The listing builds one solid part. Answer for the finished solid, in the listing's coordinates (mm). Face numbers are marked on the shaded views. A direction names the side the tool comes from. Round coordinates to 2 decimals unless told otherwise and drop trailing zeros. Loops run counter-clockwise (first coordinate to the right, second up) from the corner with the lowest first, then second, coordinate; pieces in that order, holes last. Notation, with made-up numbers: (1, 67.5) -> (45, 67.5) arc R35 ccw to (45, 106.5) -> close; hole circle Ø11 at (23, -8). An arc over 180 degrees is marked (long way). One line per question, with ' | ' between items.
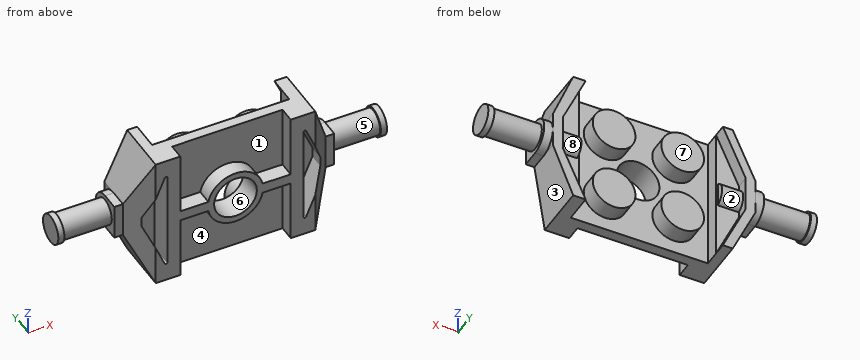
from build123d import *

# Parameters (mm, degrees)
SKETCH1_W                = 23.5
SKETCH1_H                = 15.8
BOSS_EXTRUDE1_DEPTH      = 6.3
SKETCH3_W                = 15.9
SKETCH3_H                = 15.8
CUT_EXTRUDE1_DEPTH       = 3.3
CUT_EXTRUDE2_DEPTH       = 30.009998276
CUT_EXTRUDE3_DEPTH       = 1.5
CUT_EXTRUDE4_DEPTH       = 30.009998276
BOSS_EXTRUDE2_DEPTH      = 1
BOSS_EXTRUDE3_DEPTH      = 5.6
BOSS_EXTRUDE3_DEPTH_BACK = 4.6
SKETCH9_R                = 1.5
BOSS_EXTRUDE4_START      = 1
BOSS_EXTRUDE4_DEPTH      = 1
BOSS_EXTRUDE5_DEPTH      = 5.6
BOSS_EXTRUDE5_DEPTH_BACK = 4.6
SKETCH11_R               = 1.5
CUT_EXTRUDE5_DEPTH       = 1.8
SKETCH13_R               = 2.475
CUT_EXTRUDE6_DEPTH       = 35.573689418
CUT_EXTRUDE7_DEPTH       = 2.8
SKETCH15_R               = 1.7
BOSS_EXTRUDE7_DEPTH      = 0.7
BOSS_EXTRUDE8_START      = 0.7
SKETCH16_R               = 1.7
BOSS_EXTRUDE8_DEPTH      = 0.7
SKETCH17_R               = 2.475
BOSS_EXTRUDE9_DEPTH      = 2


with BuildPart() as part:
    # Sketch1 → Boss-Extrude1 (new body)
    with BuildSketch(Plane(origin=(0, 0, 0), x_dir=(1, 0, 0), z_dir=(0, 1, 0))):
        with Locations((11.75, -7.9)):
            Rectangle(SKETCH1_W, SKETCH1_H)
    extrude(amount=BOSS_EXTRUDE1_DEPTH)

    # Sketch3 → Cut-Extrude1 (cut)
    with BuildSketch(Plane(origin=(0, 6.3, 0), x_dir=(1, 0, 0), z_dir=(0, 1, 0))):
        with Locations((11.75, -7.9)):
            Rectangle(SKETCH3_W, SKETCH3_H)
    extrude(amount=-CUT_EXTRUDE1_DEPTH, mode=Mode.SUBTRACT)

    # Sketch4 → Cut-Extrude2 (cut, through all)
    with BuildSketch(Plane(origin=(0, 6.3, 0), x_dir=(1, 0, 0), z_dir=(0, 1, 0))):
        Polygon((21.15, 0), (23.5, -5.85), (23.5, 0), align=None)
        Polygon((21.15, -15.8), (23.5, -9.95), (23.5, -15.8), align=None)
        Polygon((2.65, -15.8), (0, -9.95), (0, -15.8), align=None)
        Polygon((0, 0), (0, -5.85), (2.65, 0), align=None)
    extrude(amount=-CUT_EXTRUDE2_DEPTH, mode=Mode.SUBTRACT)

    # Sketch5 → Cut-Extrude3 (cut)
    with BuildSketch(Plane(origin=(0, 6.3, 0), x_dir=(1, 0, 0), z_dir=(0, 1, 0))):
        Polygon((3.8, 0), (1.15, -5.85), (1.15, -9.95), (3.8, -15.8), align=None)
        Polygon((19.7, 0), (19.7, -15.8), (22.35, -9.95), (22.35, -5.85), align=None)
    extrude(amount=-CUT_EXTRUDE3_DEPTH, mode=Mode.SUBTRACT)

    # Sketch7 → Cut-Extrude4 (cut, through all)
    with BuildSketch(Plane.XY.offset(15.8)):
        Polygon((0, 0), (0, 2.2), (2.65, 0), align=None)
        Polygon((21.15, 0), (23.5, 0), (23.5, 2.2), align=None)
    extrude(amount=-CUT_EXTRUDE4_DEPTH, mode=Mode.SUBTRACT)

    # Sketch8 → Boss-Extrude2 (add)
    with BuildSketch(Plane(origin=(23.5, 0, 0), x_dir=(0, 0, -1), z_dir=(1, 0, 0))):
        with BuildLine():
            Line((-9.95, 4.25), (-9.95, 2.2))
            Line((-9.95, 2.2), (-5.85, 2.2))
            Line((-5.85, 2.2), (-5.85, 4.25))
            ThreePointArc((-5.85, 4.25), (-7.9, 6.3), (-9.95, 4.25))
        make_face()
    extrude(amount=BOSS_EXTRUDE2_DEPTH)

    # Sketch9 → Boss-Extrude3 (add, two sides: drawn at the far end of the back side and taken through both)
    with BuildSketch(Plane(origin=(24.5, 0, 0), x_dir=(0, 0, -1), z_dir=(1, 0, 0)).offset(-BOSS_EXTRUDE3_DEPTH_BACK)):
        with Locations((-7.9, 4.25)):
            Circle(SKETCH9_R)
    extrude(amount=BOSS_EXTRUDE3_DEPTH + BOSS_EXTRUDE3_DEPTH_BACK)

    # Sketch10 → Boss-Extrude4 (add)
    with BuildSketch(Plane.ZY.offset(BOSS_EXTRUDE4_START)):
        with BuildLine():
            Line((5.85, 2.2), (9.95, 2.2))
            Line((9.95, 2.2), (9.95, 4.25))
            ThreePointArc((9.95, 4.25), (7.9, 6.3), (5.85, 4.25))
            Line((5.85, 4.25), (5.85, 2.2))
        make_face()
    extrude(amount=-BOSS_EXTRUDE4_DEPTH)

    # Sketch11 → Boss-Extrude5 (add, two sides: drawn at the far end of the back side and taken through both)
    with BuildSketch(Plane.ZY.offset(1).offset(-BOSS_EXTRUDE5_DEPTH_BACK)):
        with Locations(Location((7.9, 4.25, 0), (0, 0, 180))):
            Circle(SKETCH11_R)
    extrude(amount=BOSS_EXTRUDE5_DEPTH + BOSS_EXTRUDE5_DEPTH_BACK)

    # Sketch12 → Cut-Extrude5 (cut)
    with BuildSketch(Plane.XZ):
        with BuildLine():
            Line((18.3, 15.8), (5.5, 15.8))
            Line((5.5, 15.8), (5.5, 8.5))
            Line((5.5, 8.5), (8.756753271, 8.5))
            ThreePointArc((8.756753271, 8.5), (11.885259229, 11.099966048), (15.037585601, 8.528932905))
            Line((15.037585601, 8.528932905), (18.3, 8.5))
            Line((18.3, 8.5), (18.3, 15.8))
        make_face()
        with BuildLine():
            Line((8.756753271, 7.3), (5.5, 7.3))
            Line((5.5, 7.3), (5.5, 0))
            Line((5.5, 0), (18.3, 0))
            Line((18.3, 0), (18.3, 7.3))
            Line((18.3, 7.3), (15.043246729, 7.3))
            ThreePointArc((15.043246729, 7.3), (11.9, 4.7), (8.756753271, 7.3))
        make_face()
    extrude(amount=-CUT_EXTRUDE5_DEPTH, mode=Mode.SUBTRACT)

    # Sketch13 → Cut-Extrude6 (cut, through all)
    with BuildSketch(Plane.XZ):
        with Locations(Location((11.9, 7.9, 0), (0, 0, 270))):
            Circle(SKETCH13_R)
    extrude(amount=-CUT_EXTRUDE6_DEPTH, mode=Mode.SUBTRACT)

    # Sketch14 → Cut-Extrude7 (cut)
    with BuildSketch(Plane.XZ):
        with BuildLine():
            Line((4, 13.567291996), (4, 2.232708004))
            ThreePointArc((4, 2.232708004), (3.880084058, 2.085755802), (3.712067341, 2.173762423))
            Line((3.712067341, 2.173762423), (1.5, 7.35))
            Line((1.5, 7.35), (1.5, 8.45))
            Line((1.5, 8.45), (3.712067341, 13.626237577))
            ThreePointArc((3.712067341, 13.626237577), (3.880084058, 13.714244198), (4, 13.567291996))
        make_face()
        with BuildLine():
            Line((20.087932659, 2.173762423), (22.3, 7.35))
            Line((22.3, 7.35), (22.3, 8.45))
            Line((22.3, 8.45), (20.087932659, 13.626237577))
            ThreePointArc((20.087932659, 13.626237577), (19.919915942, 13.714244198), (19.8, 13.567291996))
            Line((19.8, 13.567291996), (19.8, 2.232708004))
            ThreePointArc((19.8, 2.232708004), (19.919915942, 2.085755802), (20.087932659, 2.173762423))
        make_face()
    extrude(amount=-CUT_EXTRUDE7_DEPTH, mode=Mode.SUBTRACT)

    # Sketch15 → Boss-Extrude7 (add)
    with BuildSketch(Plane.ZY.offset(6.6)):
        with Locations((7.9, 4.25)):
            Circle(SKETCH15_R)
    extrude(amount=BOSS_EXTRUDE7_DEPTH)

    # Sketch16 → Boss-Extrude8 (add)
    with BuildSketch(Plane(origin=(30.1, 0, 0), x_dir=(0, 0, -1), z_dir=(1, 0, 0)).offset(BOSS_EXTRUDE8_START)):
        with Locations(Location((-7.9, 4.25, 0), (0, 0, 180))):
            Circle(SKETCH16_R)
    extrude(amount=-BOSS_EXTRUDE8_DEPTH)

    # Sketch17 → Boss-Extrude9 (add)
    with BuildSketch(Plane(origin=(0, 3, 0), x_dir=(1, 0, 0), z_dir=(0, 1, 0))):
        with Locations(Location((7.775, -3.975, 0), (0, 0, 270))):
            Circle(SKETCH17_R)
        with Locations(Location((7.775, -11.825, 0), (0, 0, 270))):
            Circle(SKETCH17_R)
        with Locations(Location((15.725, -11.825, 0), (0, 0, 270))):
            Circle(SKETCH17_R)
        with Locations(Location((15.725, -3.975, 0), (0, 0, 270))):
            Circle(SKETCH17_R)
    extrude(amount=BOSS_EXTRUDE9_DEPTH)


solid = part.part
Q1. A cutting plane is placed at C-C on x = 16.5. Give the vertices of the cut face in (y, z), plus the area to 3 significant figures.
Numbers:
outline: (0, 7.3) -> (1.8, 7.3) -> (1.8, 0) -> (3, 0) -> (3, 1.62) -> (5, 1.62) -> (5, 6.33) -> (3, 6.33) -> (3, 9.47) -> (5, 9.47) -> (5, 14.18) -> (3, 14.18) -> (3, 15.8) -> (1.8, 15.8) -> (1.8, 8.52) -> (0, 8.52) -> close | area: 40.0 mm^2
Q2. Given pin 1 Ø1.4 at (y, z) = (4, 11.5) entering from +X; pin 2 Ø5.5 at (x, z) = (8.5, 13) entering from +Y; pin 3 Ø0.5 at (y, z) = (1.5, 14) entering from -X; pin 4 Ø6 at (x, z) = (14, 2.5) entering from -Y, each flat-ended and moving along its own axis, determine where each tip first touches the part or whether it passes through.
Numbers:
pin 1: x = 23.16 | pin 2: y = 5 | pin 3: x = 1.72 | pin 4: y = 0
Q3. Find the intervals of material crossed by line 1 (X direction, y = 2.35, z = 7.9) (3 decimals); line 2 (X direction, y = 2.5, z = 8.5); line 3 (X direction, y = 2, z = 4.25), in increasing order. Write a range as from..to.
Numbers:
line 1: -1..1.5, 4..9.425, 14.375..19.8, 22.3..24.5 | line 2: -1..1.52, 4..9.5, 14.3..19.8, 22.28..24.5 | line 3: 0.72..2.82, 4..19.8, 20.98..22.86
Q4. A cutting plane is placed at A-A on x = 11.9. Give the vertices of the cut face in (y, z) (3 decimals), plus the area to 3 significant figures.
Numbers:
outline: (0, 4.7) -> (1.8, 4.7) -> (1.8, 0) -> (3, 0) -> (3, 5.425) -> (0, 5.425) -> close; (0, 10.375) -> (3, 10.375) -> (3, 15.8) -> (1.8, 15.8) -> (1.8, 11.1) -> (0, 11.1) -> close | area: 15.6 mm^2
Q5. For a pull along Z with two mould halves and no side action, classify the marked faces 1, 2 and 3 as pulls with the +Z half, pulls with the -Z half, needs draft (parallel to the pull), parting line crosses it, or undercut.
Numbers:
face 1: needs draft | face 2: undercut | face 3: pulls with the -Z half
Q6. For the marked faces 4, 5, 6, 7 and 8, determine the directions among +Z, -Z, +X, -X, +Y, -Y from which every point of the face is accessible in a straight line to the end or side of a thin tool.
Numbers:
face 4: -Z, -Y | face 5: none | face 6: +Y, -Y | face 7: +Z, -Z, +Y | face 8: +Y
Q7. A cutting plane is placed at D-D on x = 2. Give the vertices of the cut face in (y, z).
Numbers:
outline: (0.54, 1.43) -> (6.3, 1.43) -> (6.3, 3.97) -> (4.8, 3.97) -> (4.8, 6.5) arc R1.5 ccw to (4.8, 9.3) -> (4.8, 11.83) -> (6.3, 11.83) -> (6.3, 14.37) -> (0.54, 14.37) -> (0.54, 9.62) -> (2.8, 9.62) -> (2.8, 6.18) -> (0.54, 6.18) -> close
